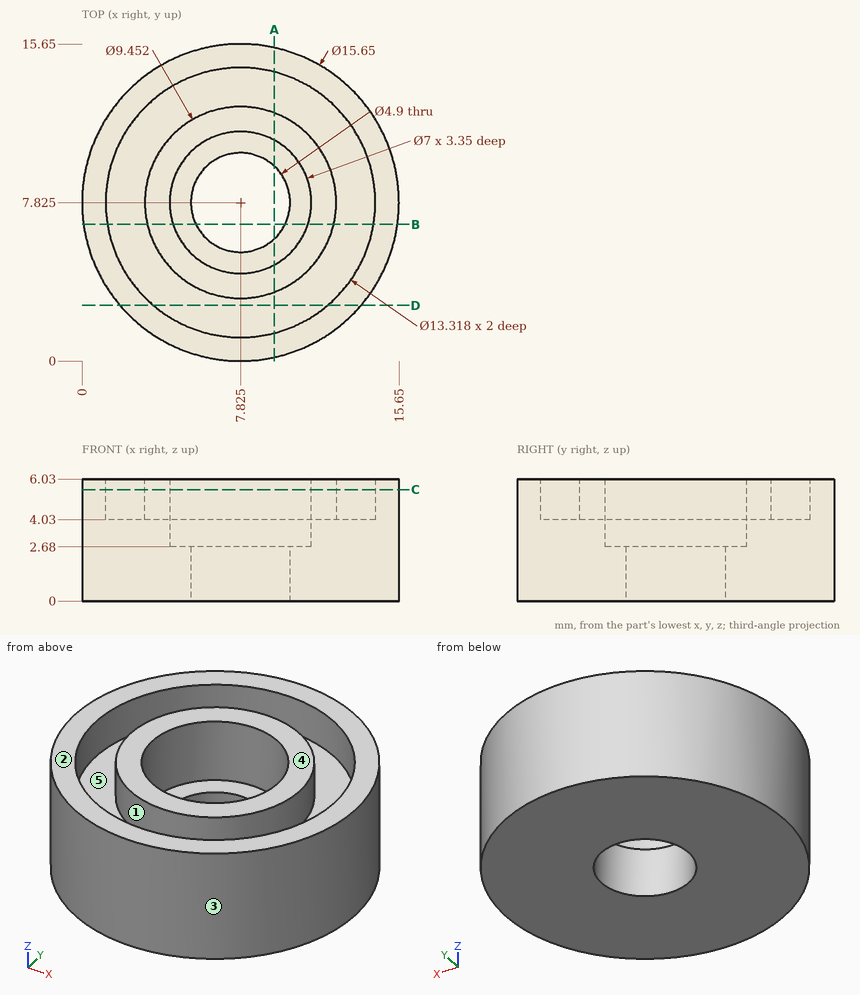
The figure shows three views and two pictorial views of one solid part (mm, origin at its lowest corner). Answer the questions. A direction names the side the tool comes from. Give positions to 0.01 mm unless a question says otherwise; leave off trailing zeros. Write each loop counter-clockwise with the first axis right and the second up, starting at its lowest first coordinate (ties: lowest second). Pieces come first, ordered by that corner, then holes. Notation, with made-up numbers: (48.25, 69) -> (94.25, 69) arc R20 cw to (94.25, 107) -> close; hole circle Ø6 at (5.5, 15). An arc over 180 degrees is marked (long way). Use one line per item in the form item = value.
1) Section A-A on x = 9.5 is taken. Write down the section's boundary in (y, z) (1 decimal).
Result:
outline = (0.2, 0) -> (6, 0) -> (6, 2.7) -> (4.8, 2.7) -> (4.8, 6) -> (3.4, 6) -> (3.4, 4) -> (1.4, 4) -> (1.4, 6) -> (0.2, 6) -> close; (9.6, 0) -> (15.5, 0) -> (15.5, 6) -> (14.3, 6) -> (14.3, 4) -> (12.2, 4) -> (12.2, 6) -> (10.9, 6) -> (10.9, 2.7) -> (9.6, 2.7) -> close
2) Section B-B on y = 6.75 is taken. Write down the section's boundary in (x, z) (1 decimal).
Result:
outline = (0.1, 0) -> (5.6, 0) -> (5.6, 2.7) -> (4.5, 2.7) -> (4.5, 6) -> (3.2, 6) -> (3.2, 4) -> (1.3, 4) -> (1.3, 6) -> (0.1, 6) -> close; (10, 0) -> (15.6, 0) -> (15.6, 6) -> (14.4, 6) -> (14.4, 4) -> (12.4, 4) -> (12.4, 6) -> (11.2, 6) -> (11.2, 2.7) -> (10, 2.7) -> close
3) Straight lines are drawn through the part: probe 1 along X at (y, z) = (5.25, 5) (1 decimal); probe 2 along Y at (x, z) = (3, 5.75) (1 decimal); probe 3 along Z at (x, y) = (12.75, 7.5). For each, find the intervals that lie inside material, in ascending order.
Result:
probe_1 = 0.4 to 1.7, 3.9 to 5.5, 10.2 to 11.8, 14 to 15.2
probe_2 = 1.7 to 3.2, 12.4 to 14
probe_3 = 0 to 4.03
4) For a pull along Y with two mould halves and no side action, classify the marked faces 3, 4 and 5 as +Y half, -Y half, draft (parallel to the pull), parting line (faces both ways), or undercut.
Result:
face_3 = parting line
face_4 = draft
face_5 = undercut
5) A tool of negligible diameter and unlimited length cuts with its end or side. For the marked faces 1 and 2, from which of +Z, -Z, +X, -X, +Y, -Y can it reach the whole face along a straight path? Write none if from no direction.
Result:
face_1 = +Z
face_2 = +Z, +X, -X, +Y, -Y
6) Section D-D on y = 2.75 is taken. Write down the section's boundary in (x, z).
Result:
outline = (1.87, 0) -> (13.78, 0) -> (13.78, 6.03) -> (12.14, 6.03) -> (12.14, 4.03) -> (3.51, 4.03) -> (3.51, 6.03) -> (1.87, 6.03) -> close
7) Each of these flat-tipped pins is pushed along its axis until it touches: P1, Ø4, axis at x = 5.5, y = 7, coming from the +Z side; P2, Ø6.5, axis at x = 7.825, y = 7.825, coming from the +Z side; P3, Ø3, axis at x = 4, z = 1, coming from the -Y side; P4, Ø1, axis at y = 9, z = 1.5, coming from the +X side. Where does it stop, or does it pass through?
Result:
P1 = 6.03
P2 = 2.68
P3 = 0.35
P4 = 15.62
8) Section C-C on z = 5.5 is taken. Count the separate pieces of the cut face and the enclosed holes in it.
Result:
separate_pieces = 2
enclosed_holes = 2
